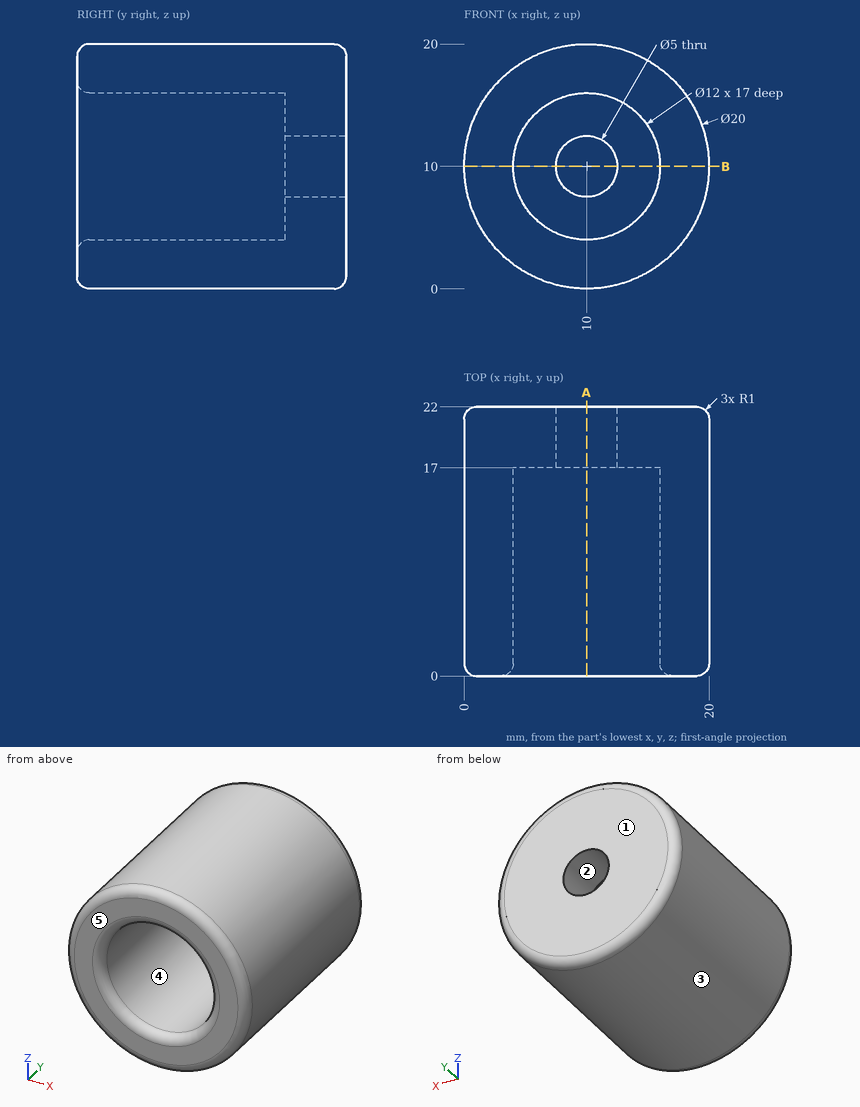
Geometry check sheet. Reference: drawing and pictorial views, mm from the part's lowest x, y, z. A direction names the side the tool comes from. Give positions to 0.01 mm unless a question says otherwise; leave off trailing zeros. Write each loop counter-clockwise with the first axis right and the second up, starting at its lowest first coordinate (ties: lowest second). Pieces come first, ordered by that corner, then holes. Notation, with made-up numbers: (54, -35.5) -> (99, -35.5) arc R18 ccw to (99, -3.5) -> close; hole circle Ø9 at (37, -17.75). An arc over 180 degrees is marked (long way). One line per item, written item: value. Start each with the question number.
Item 1: Gauge pin test, flat ends, axial feed: pin 1 (10 mm diameter, centred on y = 13.5, z = 3.5, fed in from +X); pin 2 (6 mm diameter, centred on y = 17.5, z = 5, fed in from -X); pin 3 (1 mm diameter, centred on x = 12.5, z = 7.5, fed in from -Y). Record the tip position at first contact, or that the pin passes through.
Item 2: Material ranges on probe 1 along X at (y, z) = (10.75, 10); probe 2 along Z at (x, y) = (10, 20.85); probe 3 along Y at (x, z) = (5.5, 6.25), recorded low to high. Write a range as from..to.
Item 3: Section check B-B on z = 10. Record the cut outline in (x, y), then the cut area to 3 significant figures.
Item 4: Draft check along Z on the marked faces 1, 2 and 3. Enter one of: +Z half, -Z half, draft (parallel to the pull), parting line (faces both ways), or undercut.
Item 5: Section check A-A on x = 10. Record the cut outline in (y, z).
Item 6: Tool access check on the marked faces 4 and 5. Record the directions out of +Z, -Z, +X, -X, +Y, -Y that give a thin tool (end or side, any length) a straight path to the whole face; none if there is none.
Results list:
1. pin 1: x = 19.89
1. pin 2: x = 0.2
1. pin 3: y = 17
2. probe 1: 0..4, 16..20
2. probe 2: 0..7.5, 12.5..20
2. probe 3: 17..22
3. outline: (0, 1) arc R1 ccw to (1, 0) -> (3, 0) arc R1 ccw to (4, 1) -> (4, 17) -> (7.5, 17) -> (7.5, 22) -> (1, 22) arc R1 ccw to (0, 21) -> close; (12.5, 17) -> (16, 17) -> (16, 1) arc R1 ccw to (17, 0) -> (19, 0) arc R1 ccw to (20, 1) -> (20, 21) arc R1 ccw to (19, 22) -> (12.5, 22) -> close
3. area: 210 mm²
4. face 1: draft
4. face 2: undercut
4. face 3: parting line
5. outline: (0, 1) arc R1 ccw to (1, 0) -> (21, 0) arc R1 ccw to (22, 1) -> (22, 7.5) -> (17, 7.5) -> (17, 4) -> (1, 4) arc R1 ccw to (0, 3) -> close; (0, 17) arc R1 ccw to (1, 16) -> (17, 16) -> (17, 12.5) -> (22, 12.5) -> (22, 19) arc R1 ccw to (21, 20) -> (1, 20) arc R1 ccw to (0, 19) -> close
6. face 4: -Y
6. face 5: +Z, -Z, +X, -X, -Y
